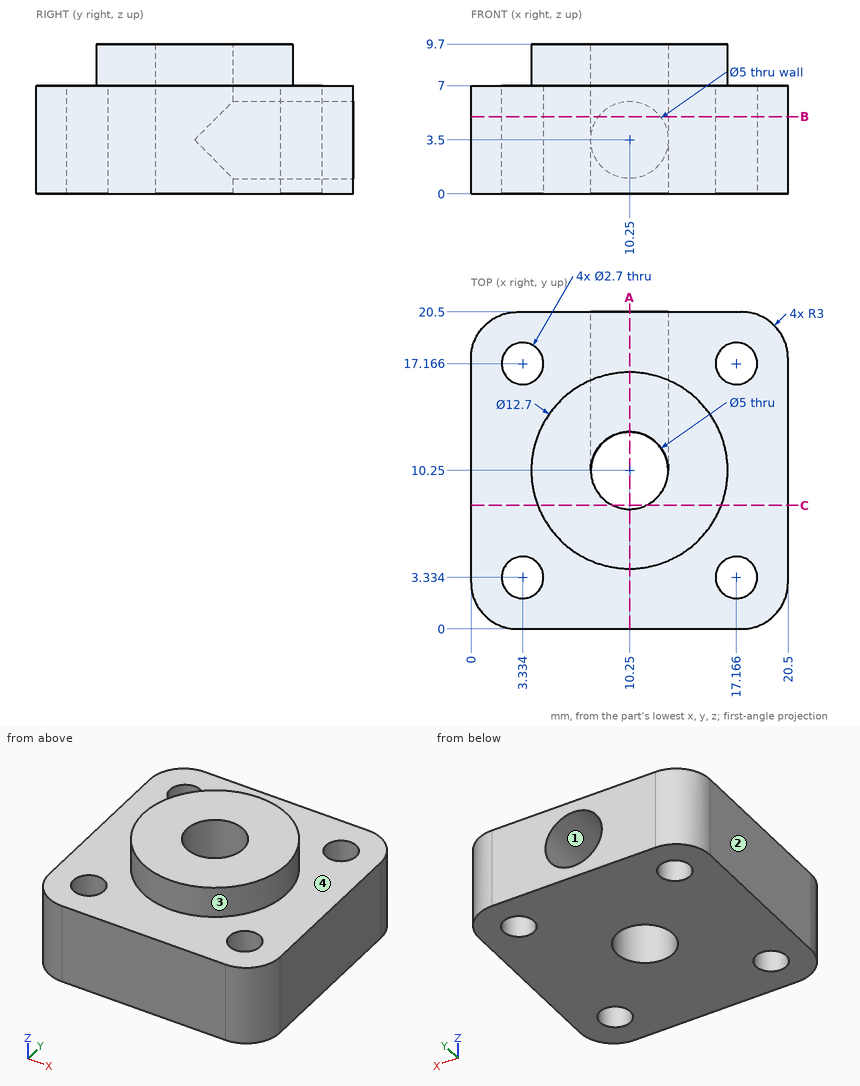
Drawing for the job (mm, zero at the part's lowest x, y, z). Round coordinates to 2 decimals unless told otherwise and drop trailing zeros. Order: outer loops, then holes, each group sorted by start corner. A loop starts at its lowest first (then second) coordinate and runs counter-clockwise, first axis right, second up.
Item 1: Pin check, flat tips, straight feed: pin 1 (2.5 mm diameter, centred on x = 17.17, y = 3.33, fed in from +Z); pin 2 (3 mm diameter, centred on x = 10.25, z = 3.5, fed in from +Y); pin 3 (3 mm diameter, centred on x = 16, y = 2.5, fed in from +Z). Stop position of each tip, or through.
Item 2: Saw through at B-B on z = 5. State how many separate pieces and enclosed holes the cut face has, then the cut area to 3 significant figures.
Item 3: Saw through at C-C on y = 8. Write the cut outline in (x, z).
Item 4: Probe line 1 along X through (y, z) = (15.5, 3.5); line 2 along X through (y, z) = (16.25, 2.5) (1 decimal); line 3 along Z through (x, y) = (16.25, 18.5). List the from-to ranges inside material, lowest first.
Item 5: Saw through at A-A on x = 10.25. Write the cut outline in (y, z).
Item 6: Mould opens along X. For the marked faces 1, 2, 3 and 4 say: pulls with the +X half, pulls with the -X half, needs draft (parallel to the pull), parting line crosses it, or undercut.
Reported:
1. pin 1: passes through
1. pin 2: stops at y = 8.25
1. pin 3: stops at z = 7
2. separate pieces: 1
2. enclosed holes: 4
2. area: 338 mm2
3. outline: (0, 0) - (9.16, 0) - (9.16, 9.7) - (4.31, 9.7) - (4.31, 7) - (0, 7) - close; (11.34, 0) - (20.5, 0) - (20.5, 7) - (16.19, 7) - (16.19, 9.7) - (11.34, 9.7) - close
4. line 1: x = 0 to 7.75, 12.75 to 20.5
4. line 2: x = 0 to 2.3, 4.3 to 8, 12.5 to 16.2, 18.2 to 20.5
4. line 3: z = 0 to 7
5. outline: (0, 0) - (7.75, 0) - (7.75, 9.7) - (3.9, 9.7) - (3.9, 7) - (0, 7) - close; (12.75, 0) - (20.5, 0) - (20.5, 1) - (12.75, 1) - close; (12.75, 6) - (20.5, 6) - (20.5, 7) - (16.6, 7) - (16.6, 9.7) - (12.75, 9.7) - close
6. face 1: undercut
6. face 2: pulls with the -X half
6. face 3: parting line crosses it
6. face 4: needs draft
